Verification items for this drawing (mm, ordinates from the low corner). Coordinates: 2 decimals unless noted, no trailing zeros. Order: outer loops, then holes, each group sorted by start corner. A loop starts at its lowest first (then second) coordinate and runs counter-clockwise, first axis right, second up. Notation, with made-up numbers: M 83,6 L 107,6 A10 cw 107,12 Z; hole C -16.5,-22 d1. An arc over 180 degrees is marked long. One line per item, written item: value. Start each with the question number.
1) Go/stop test with flat-tipped pins: P1, Ø1.5, axis at y = 3, z = 84, coming from the -X side; P2, Ø9, axis at x = 47.5, y = 9.5, coming from the -Z side; P3, Ø3, axis at x = 352, z = 13.5, coming from the -Y side; P4, Ø21, axis at x = 66, z = 34.5, coming from the -Y side. Record where each tip stops, or that it passes through.
2) Thickness scan on L1, parallel to Y at x = 70, z = 53; L2, parallel to X at y = 9.5, z = 12; L3, parallel to X at y = 3.75, z = 21. Record the ranges inside material, lowest first. Write a range as from..to.
3) Sectioned sample at A-A, the plane y = 2.25. Enter the section's corners in (x, z).
4) Sectioned sample at B-B, the plane z = 35.5. Enter the section's corners in (x, y).
5) Sectioned sample at C-C, the plane z = 7. Enter the section's corners in (x, y).
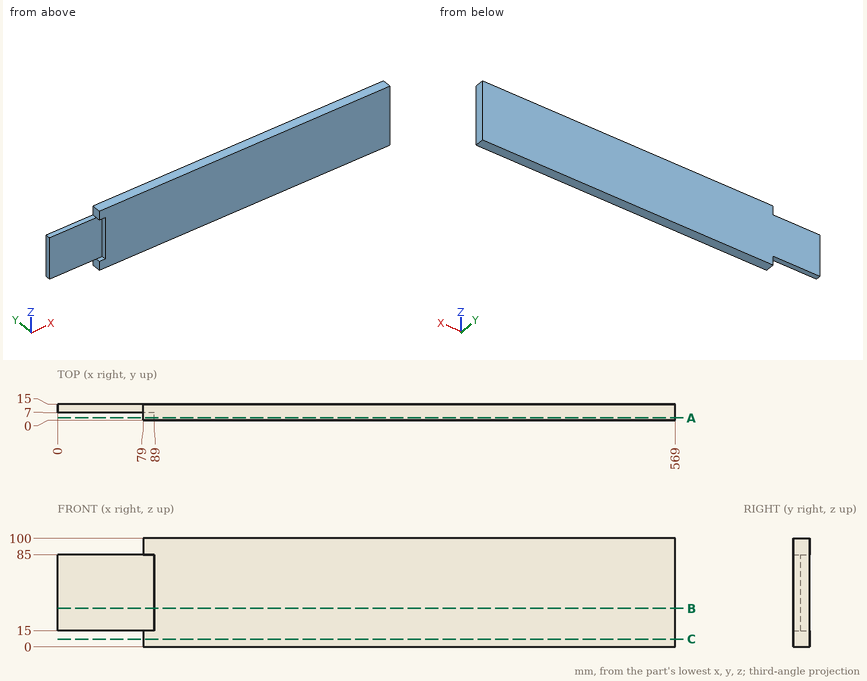
Final values:
1. P1: stops at x = 89
1. P2: stops at z = 15
1. P3: stops at y = 0
1. P4: stops at y = 7
2. L1: y = 7..15
2. L2: x = 79..569
2. L3: x = 89..569
3. outline: M 79,0 L 569,0 L 569,100 L 79,100 L 79,85 L 89,85 L 89,15 L 79,15 Z
4. outline: M 0,7 L 89,7 L 89,0 L 569,0 L 569,15 L 0,15 Z
5. outline: M 79,0 L 569,0 L 569,15 L 79,15 Z
